Input: dimensioned drawing with shaded views. Units: mm. Origin: part minimum x, y, z. Round coordinates to 2 decimals unless told otherwise and drop trailing zeros. Loops run counter-clockwise (first coordinate to the right, second up) from the corner with the lowest first, then second, coordinate; pieces in that order, holes last. Notation, with made-up numbers: (70.25, -3) - (114.25, -3) arc R13 cw to (114.25, 15) - close; hole circle Ø4 at (74, -12.75). An arc over 180 degrees is marked (long way). One line per question, with ' | ' between items. Start each with the question number.
1. Pin query (flat end, axial travel): pin 1 (6 mm diameter, centred on y = 49.5, z = 1.5, fed in from +X); pin 2 (1 mm diameter, centred on y = 97.5, z = 8, fed in from -X); pin 3 (2 mm diameter, centred on x = 1.5, z = 7, fed in from +Y). Return the tip coordinate at first contact, or that it passes through.
2. Cut plane A-A (y = 86). Return loops of the section in (x, z).
3. Ray query, line 1 (Z direction, x = 5.5, y = 109); line 2 (Y direction, x = 2, z = 8.75); line 3 (Z direction, x = 7.25, y = 147). Return the intervals inside material, ascending.
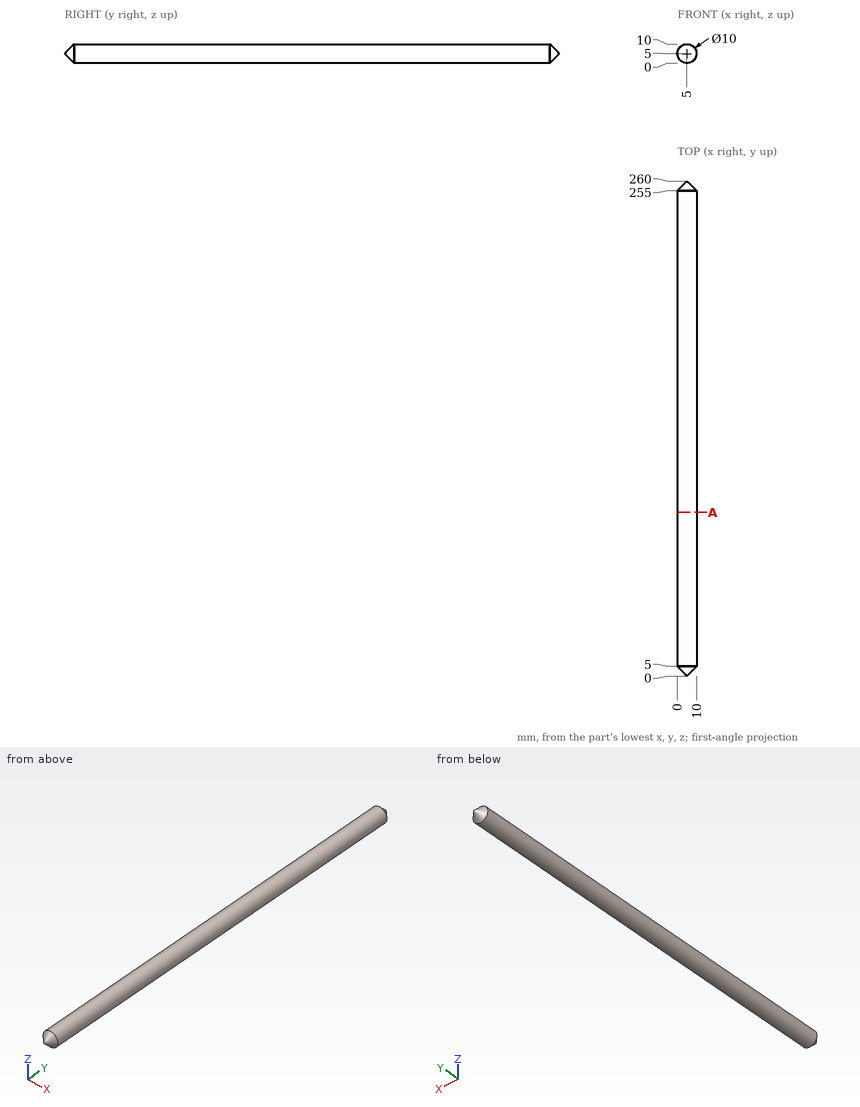
Answers follow:
1) pin 1: stops at x = 9.97 | pin 2: stops at x = 0.67 | pin 3: stops at y = 256.97
2) outline: circle Ø10 at (5, 5)
3) line 1: z = 0.03 to 9.97 | line 2: y = 4.8 to 255.2 | line 3: z = 0.53 to 9.47
